from build123d import *

# Parameters (mm, degrees)
SKETCH1_W           = 47.5
SKETCH1_H           = 73
BOSS_EXTRUDE1_DEPTH = 22
CUT_EXTRUDE1_DEPTH  = 18
SKETCH4_R           = 2
CUT_EXTRUDE2_DEPTH  = 18
SKETCH5_W           = 5
SKETCH5_H           = 2.5
CUT_EXTRUDE3_DEPTH  = 6.5
SKETCH9_W           = 5
SKETCH9_H           = 2.5
CUT_EXTRUDE4_DEPTH  = 6.5


with BuildPart() as part:
    # Sketch1 → Boss-Extrude1 (new body)
    with BuildSketch(Plane(origin=(0, 0, 0), x_dir=(1, 0, 0), z_dir=(0, 1, 0))):
        with Locations((-33.624481527, 0.818123821)):
            Rectangle(SKETCH1_W, SKETCH1_H)
    extrude(amount=BOSS_EXTRUDE1_DEPTH)

    # Sketch2 → Cut-Extrude1 (cut)
    with BuildSketch(Plane.XZ):
        Polygon((-57.374481527, 27.681876179), (-50.374481527, 27.681876179), (-50.374481527, 35.681876179), (-13.874481527, 35.681876179), (-13.874481527, 27.681876179), (-9.874481527, 27.681876179), (-9.874481527, -29.318123821), (-16.874481527, -29.318123821), (-16.874481527, -37.318123821), (-53.374481527, -37.318123821), (-53.374481527, -29.318123821), (-57.374481527, -29.318123821), align=None)
    extrude(amount=-CUT_EXTRUDE1_DEPTH, mode=Mode.SUBTRACT)

    # Sketch4 → Cut-Extrude2 (cut)
    with BuildSketch(Plane.XZ):
        with Locations(Location((-53.374481527, 31.681876179, 0), (0, 0, 270))):
            Circle(SKETCH4_R)
        with Locations(Location((-13.874481527, -33.318123821, 0), (0, 0, 270))):
            Circle(SKETCH4_R)
    extrude(amount=-CUT_EXTRUDE2_DEPTH, mode=Mode.SUBTRACT)

    # Sketch5 → Cut-Extrude3 (cut)
    with BuildSketch(Plane.ZY.offset(57.374481527)):
        with Locations((31.798626617, 3.25)):
            Rectangle(SKETCH5_W, SKETCH5_H)
    extrude(amount=-CUT_EXTRUDE3_DEPTH, mode=Mode.SUBTRACT)

    # Sketch9 → Cut-Extrude4 (cut)
    with BuildSketch(Plane(origin=(-9.874481527, 0, 0), x_dir=(0, 0, -1), z_dir=(1, 0, 0))):
        with Locations((33.394669179, 3.25)):
            Rectangle(SKETCH9_W, SKETCH9_H)
    extrude(amount=-CUT_EXTRUDE4_DEPTH, mode=Mode.SUBTRACT)


solid = part.part
Geometry check sheet. Reference: the model listing, model coordinates, mm. A direction names the side the tool comes from. Round coordinates to 2 decimals unless told otherwise and drop trailing zeros. Loops run counter-clockwise (first coordinate to the right, second up) from the corner with the lowest first, then second, coordinate; pieces in that order, holes last. Notation, with made-up numbers: (-38, 31.5) - (14, 31.5) arc R18 ccw to (14, 43.5) - close; hole circle Ø3 at (51.5, -14). An arc over 180 degrees is marked (long way). Answer as CSV lines item,"result".
(1) Depth check by flat-ended pin: pin 1 Ø1.5 at (x, z) = (-13.5, -33) entering from -Y; pin 2 Ø2 at (x, y) = (-15, 6) entering from +Z. Enter the tip coordinate at first touch or a pass-through.
Output values:
pin 1,"stops at y = 18"
pin 2,"stops at z = -29.32"
(2) Set-up check for faces 5 (the face through (-54, 9, 27.682)), 6 (the face through (-34, 18.2, 35.682)), 7 (the face through (-33, 18, 0)), 8 (the face through (-50.374, 9, 32)), 9 (the face through (-16.374, 3, -33)): record each of +Z, -Z, +X, -X, +Y, -Y from which the full face is reachable in a straight line by a thin tool's end or side.
Output values:
face 5,"+X, -X, -Y"
face 6,"+Z, +X, -X, +Y, -Y"
face 7,"-Y"
face 8,"+Z, -Z, -Y"
face 9,"+X"
(3) Cross-section at C-C, the plane z = 0. Enter the section's corners in (x, y).
Output values:
outline,"(-57.37, 18) - (-9.87, 18) - (-9.87, 22) - (-57.37, 22) - close"
(4) Material ranges on line 1 along X through (y, z) = (14.5, -29.5); line 2 along X through (y, z) = (6.5, 32); line 3 along X through (y, z) = (11, 32.5), recorded low to high.
Output values:
line 1,"x = -57.37 to -53.37, -16.87 to -9.87"
line 2,"x = -57.37 to -55.35, -51.4 to -50.37, -13.87 to -9.87"
line 3,"x = -57.37 to -55.2, -51.55 to -50.37, -13.87 to -9.87"
(5) Cross-section at B-B, the plane x = -35. Enter the section's corners in (y, z).
Output values:
outline,"(18, -37.32) - (22, -37.32) - (22, 35.68) - (18, 35.68) - close"
(6) Cross-section at A-A, the plane y = 8. Enter the section's corners in (x, z), and give its area (3 significant figures).
Output values:
outline,"(-57.37, -37.32) - (-53.37, -37.32) - (-53.37, -29.32) - (-57.37, -29.32) - close; (-57.37, 27.68) - (-50.37, 27.68) - (-50.37, 35.68) - (-57.37, 35.68) - close; (-16.87, -37.32) - (-9.87, -37.32) - (-9.87, -29.32) - (-16.87, -29.32) - close; (-13.87, 27.68) - (-9.87, 27.68) - (-9.87, 35.68) - (-13.87, 35.68) - close; hole circle Ø4 at (-53.37, 31.68); hole circle Ø4 at (-13.87, -33.32)"
area,"151 mm²"
(7) Release check for a two-part mould opening along X. For faces 1 (the face through (-57.374, 18.2, -0.3)), 2 (the face through (-53, 18, 32)), 3 (the face through (-53.374, 9, -33)), 4 (the face through (-11.6, 2, -33.4)) record: released by +X, released by -X, zero draft, split by the parting line, or undercut.
Output values:
face 1,"released by -X"
face 2,"undercut"
face 3,"undercut"
face 4,"zero draft"
